Here's how the part is built. I have some questions about the finished solid (model axes, mm). A direction names the side the tool comes from. Coordinates: 2 decimals unless noted, no trailing zeros. Write each loop counter-clockwise with the first axis right and the second up, starting at its lowest first coordinate (ties: lowest second). Pieces come first, ordered by that corner, then holes. Notation, with made-up numbers: (-28, 86.5) -> (-3, 86.5) arc R20 ccw to (-3, 92.5) -> close; hole circle Ø8 at (-21.75, 45.25). An arc over 180 degrees is marked (long way). Put each result on its own line as item: value. Start each with the question number.
Item 1: For pin 1 (1.2 mm diameter, centred on x = 7.5, z = -18.5, fed in from -Y); pin 2 (1.5 mm diameter, centred on x = 1.5, z = 4, fed in from -Y); pin 3 (2.5 mm diameter, centred on x = 24.43, z = 26.03, fed in from -Y); pin 4 (2 mm diameter, centred on x = 30, y = 1, fed in from -Z), each with a flat end and sliding along its axis, tell me the tip position at first contact or that it passes through.
Item 2: I want a section at D-D, the plane z = 5.5. List the corners of the cut face in (x, y) for me, then the cut area to 3 significant figures.
Item 3: On a 3-axis mill with a long thin cutter (end or side, diameter ignored), from which of +Z, -Z, +X, -X, +Y, -Y can I reach the whole of each face in a straight line? I mean faces 1 (the face through (30, 1, -16.463)), 2 (the face through (-9, 1, -16.463)), 3 (the face through (11, 3.2, -17)). Say none if no direction works.
Item 4: I need wall thicknesses on line 1 (Z direction, x = 26.5, y = 3.05); line 2 (Z direction, x = 3.5, y = 1.7); line 3 (X direction, y = 2.6, z = -7). Which ranges of each line are inside material? Lowest first, please. Write a range as [from, to].
Item 5: I want a section at B-B, the plane x = -2.5. List the corners of the cut face in (y, z) for me.
Item 6: If we mould it in two halves opening along Z, with no side actions, what happens to faces 4 (the face through (-9.22, 2.03, -22.89)), 5 (the face through (-3.44, 2.78, 24.44)), 6 (the face through (16.462, 3, 31))? For each: released by +Z, released by -Z, zero draft, split by the parting line, or undercut.
Item 7: I want a section at A-A, the plane z = -14.5. List the corners of the cut face in (x, y) for me, then the cut area to 3 significant figures.
from build123d import *

# Parameters (mm, degrees)
SKETCH1_R           = 1.5875000000000004
SKETCH1_R_2         = 1.5874999999999988
SKETCH1_R_3         = 1.5874999999999977
SKETCH1_R_4         = 1.5874999999999986
BOSS_EXTRUDE2_DEPTH = 4
CUT_EXTRUDE1_DEPTH  = 1.6
CUT_EXTRUDE2_DEPTH  = 1.6002
SKETCH4_W           = 2
SKETCH4_H           = 5
SKETCH4_W_2         = 2.000000000000001
CUT_EXTRUDE3_DEPTH  = 2.5
CUT_EXTRUDE4_DEPTH  = 3
FILLET1_R           = 2
FILLET2_R           = 1


with BuildPart() as part:
    # Sketch1 → Boss-Extrude2 (new body)
    with BuildSketch(Plane(origin=(0, 0, 0), x_dir=(1, 0, 0), z_dir=(0, 1, 0))):
        Polygon((-9.817707317102446, 23.463272745610922), (30.74229268289756, 23.463272745610926), (30.742292682897567, -32.336727254389075), (-9.81770731710244, -32.336727254389075), align=None)
        with Locations(Location((-3.5077073171024433, 6.993272745610932, 0), (0, 0, 270))):
            Circle(SKETCH1_R, mode=Mode.SUBTRACT)
        with Locations(Location((24.432292682897558, 6.993272745610931, 0), (0, 0, 270))):
            Circle(SKETCH1_R_2, mode=Mode.SUBTRACT)
        with Locations(Location((-3.5077073171024393, -26.026727254389073, 0), (0, 0, 270))):
            Circle(SKETCH1_R_3, mode=Mode.SUBTRACT)
        with Locations(Location((24.432292682897558, -26.026727254389073, 0), (0, 0, 270))):
            Circle(SKETCH1_R_4, mode=Mode.SUBTRACT)
    extrude(amount=BOSS_EXTRUDE2_DEPTH)

    # Sketch1<4> → Cut-Extrude1 (cut)
    with BuildSketch(Plane(origin=(0, 0, 0), x_dir=(1, 0, 0), z_dir=(0, 1, 0))):
        Polygon((-7.817707317102445, 21.463272745610922), (28.742292682897556, 21.463272745610926), (28.742292682897563, -30.336727254389075), (-7.817707317102438, -30.336727254389075), align=None)
    extrude(amount=CUT_EXTRUDE1_DEPTH, mode=Mode.SUBTRACT)

    # Sketch3 → Cut-Extrude2 (cut)
    with BuildSketch(Plane.XZ.offset(-1.6)):
        Polygon((-7.317707317102444, -15.463272745610924), (28.242292682897553, -15.463272745610924), (28.242292682897553, -19.463272745610922), (-7.317707317102443, -19.463272745610922), align=None)
        Polygon((2.182292682897542, 28.33672725438907), (18.74229268289756, 28.33672725438907), (18.74229268289756, 18.336727254389068), (2.1822926828975433, 18.336727254389068), align=None)
        Polygon((4.182292682897542, 16.336727254389075), (27.242292682897556, 16.336727254389075), (27.242292682897556, 2.3367272543890727), (4.182292682897544, 2.3367272543890727), align=None)
    extrude(amount=-CUT_EXTRUDE2_DEPTH, mode=Mode.SUBTRACT)

    # Sketch4 → Cut-Extrude3 (cut)
    with BuildSketch(Plane.XZ):
        with Locations((29.74229268289756, -18.96327274561092)):
            Rectangle(SKETCH4_W, SKETCH4_H)
        with Locations((-8.817707317102446, -18.96327274561092)):
            Rectangle(SKETCH4_W_2, SKETCH4_H)
    extrude(amount=-CUT_EXTRUDE3_DEPTH, mode=Mode.SUBTRACT)

    # Sketch5 → Cut-Extrude4 (cut)
    with BuildSketch(Plane(origin=(0, 0, 32.336727254389075), x_dir=(-1, 0, 0), z_dir=(0, 0, -1))):
        Polygon((-16.462292682897562, 4.000000000000003), (-4.462292682897565, 4.000000000000007), (-4.462292682897558, -5.590997478767573), (-16.462292682897562, -5.590997478767577), align=None)
    extrude(amount=CUT_EXTRUDE4_DEPTH, mode=Mode.SUBTRACT)

    # Fillet1
    fillet1_edges = [part.edges().sort_by_distance(p)[0] for p in [
        (-9.817707317102446, 2, -23.463272745610922),
        (30.74229268289756, 2, -23.463272745610926),
        (30.742292682897567, 2, 32.336727254389075),
        (-9.81770731710244, 2, 32.336727254389075),
    ]]
    fillet(fillet1_edges, radius=FILLET1_R)

    # Fillet2
    fillet2_edges = [part.edges().sort_by_distance(p)[0] for p in [
        (10.46229268289756, 1.6, 29.336727254389075),
        (4.462292682897564, 1.6, 29.836727254389075),
        (16.462292682897562, 1.6000000000000003, 29.836727254389075),
        (16.462292682897562, 2.000000000000001, 32.336727254389075),
        (4.462292682897563, 2.0000000000000036, 32.336727254389075),
        (16.462292682897562, 0, 31.336727254389075),
        (4.462292682897562, 0, 31.336727254389075),
    ]]
    fillet(fillet2_edges, radius=FILLET2_R - 0.0001)  # a hair under: the kernel refuses the full size


solid = part.part
Calculated:
1. pin 1: stops at y = 3.2
1. pin 2: stops at y = 1.6
1. pin 3: passes through
1. pin 4: stops at z = -23.45
2. outline: (-9.82, 0) -> (-7.82, 0) -> (-7.82, 1.6) -> (4.18, 1.6) -> (4.18, 3.2) -> (27.24, 3.2) -> (27.24, 1.6) -> (28.74, 1.6) -> (28.74, 0) -> (30.74, 0) -> (30.74, 4) -> (-9.82, 4) -> close
2. area: 66.8 mm2
3. face 1: +X, -Y
3. face 2: -X, -Y
3. face 3: -Y
4. line 1: z = [-23.46, -19.46], [-15.46, 2.34], [16.34, 32.34]
4. line 2: z = [-23.46, -19.46], [-15.46, 18.34], [28.34, 32.34]
4. line 3: x = [-9.82, -5.1], [-1.92, 22.84], [26.02, 30.74]
5. outline: (0, -23.46) -> (4, -23.46) -> (4, -8.22) -> (1.6, -8.22) -> (1.6, -15.46) -> (3.2, -15.46) -> (3.2, -19.46) -> (1.6, -19.46) -> (1.6, -21.46) -> (0, -21.46) -> close; (0, 30.34) -> (1.6, 30.34) -> (1.6, 27.25) -> (4, 27.25) -> (4, 32.34) -> (0, 32.34) -> close; (1.6, -5.77) -> (4, -5.77) -> (4, 24.8) -> (1.6, 24.8) -> close
6. face 4: released by -Z
6. face 5: undercut
6. face 6: zero draft
7. outline: (-9.82, 0) -> (-7.82, 0) -> (-7.82, 1.6) -> (28.74, 1.6) -> (28.74, 0) -> (30.74, 0) -> (30.74, 4) -> (-9.82, 4) -> close
7. area: 104 mm2
